from build123d import *

# Parameters (mm, degrees)
F1_DEPTH = 8.3
F2_R     = 1.55
F3_DEPTH = 23.001
F4_R     = 1.55
F5_DEPTH = 16.001
F6_R     = 4.14999


# Not quite as in the source:
# - a fillet or chamfer is up to 0.001 mm smaller than in the source, because OpenCascade refuses the exact size


with BuildPart() as f1:
    # F0 (on Top) → F1 (new body)
    with BuildSketch(Plane.XY):
        Polygon((-57.5197213515, -7.7541078215), (-65.8197213515, -7.7541078215), (-65.8197213515, -14.7041078215), (-49.7500874824, -14.7041078215), (-49.7500874824, -7.7041078215), (-41.4500874824, -7.7041078215), (-41.4500874824, 1.2958921785), (-49.7500874824, 1.2958921785), (-49.7500874824, 8.2958921785), (-65.8197213515, 8.2958921785), (-65.8197213515, 1.3458921785), (-57.5197213515, 1.3458921785), align=None)
    extrude(amount=F1_DEPTH)

    # F2 (on face) → F3 (cut, through all)
    with BuildSketch(Plane.XZ.offset(14.7041078215)):
        with Locations((-61.6697213515, 4.15)):
            Circle(F2_R)
    extrude(amount=-F3_DEPTH, mode=Mode.SUBTRACT)

    # F4 (on face) → F5 (cut, through all)
    with BuildSketch(Plane.XZ.offset(7.7041078215)):
        with Locations((-45.6000874824, 4.15)):
            Circle(F4_R)
    extrude(amount=-F5_DEPTH, mode=Mode.SUBTRACT)

    # F6 (radius 4.15 in the source; OpenCascade refuses exactly that, so slightly less here)
    f6_edges = [f1.edges().sort_by_distance(p)[0] for p in [
        (-65.819721, 4.820892, 8.3),
        (-65.819721, 4.820892, 0),
        (-65.819721, -11.229108, 0),
        (-65.819721, -11.229108, 8.3),
        (-41.450087, -3.204108, 0),
        (-41.450087, -3.204108, 8.3),
    ]]
    fillet(f6_edges, radius=F6_R)


solid = f1.part
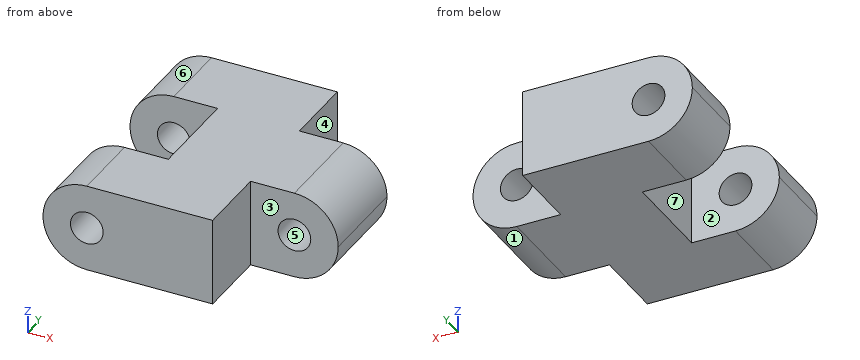
Could you check a few things on this model? Use its own coordinates, in mm. Face numbers are marked on the shaded views. A direction names the side the tool comes from. Coordinates: 2 decimals unless noted, no trailing zeros. Write each loop counter-clockwise with the first axis right and the second up, starting at its lowest first coordinate (ties: lowest second). Pieces come first, ordered by that corner, then holes. Notation, with made-up numbers: (51.5, 59.25) - (79.5, 59.25) arc R24 ccw to (79.5, 69.25) - close; hole circle Ø1 at (88, 62). An arc over 180 degrees is marked (long way). Put each result on its own line as item: value. Start each with the question number.
Q1. I want a section at B-B on z = 5. Write out the boundary of the cut face in (x, y).
Q2. I'm going to push flat-ended pins straight in: P1, Ø2, axis at x = -47, z = 6.5, coming from the -Y side; P2, Ø2.5, axis at x = -47, z = 2.5, coming from the +Y side; P3, Ø1.5, axis at y = 4, z = 6.5, coming from the -X side. Where does each tip first touch, or does it pass through?
Q3. Which directions (+Z, -Z, +X, -X, +Y, -Y) give clear straight access to the entire face, cutting with the end or side of a thin tool? Please do the marked faces 1, 2, 3 and 4.
Q4. I want a section at C-C on x = -62.25. Write out the boundary of the cut face in (y, z), plus the area to 3 significant figures.
Q5. Please list where these lines run through material, in increasing order: L1, parallel to Y at x = -63, z = 2; L2, parallel to X at y = -9, z = 4; L3, parallel to Y at x = -45.75, z = 6.
Q6. I want a section at D-D on x = -44.75. Write out the boundary of the cut face in (y, z), plus the area to 3 significant figures.
Q7. Thinking about a two-plate mould opening in Z: for the marked faces 5, 6 and 7, which applies, pulls with the +Z half, pulls with the -Z half, needs draft (parallel to the pull), parting line crosses it, or undercut?
Checks:
1. outline: (-65.73, -14.7) - (-62.97, -14.7) - (-62.97, -7.75) - (-65.73, -7.75) - close; (-65.73, 1.35) - (-62.97, 1.35) - (-62.97, 8.3) - (-65.73, 8.3) - close; (-60.37, -14.7) - (-49.75, -14.7) - (-49.75, -7.7) - (-46.9, -7.7) - (-46.9, 1.3) - (-49.75, 1.3) - (-49.75, 8.3) - (-60.37, 8.3) - (-60.37, 1.35) - (-57.52, 1.35) - (-57.52, -7.75) - (-60.37, -7.75) - close; (-44.3, -7.7) - (-41.54, -7.7) - (-41.54, 1.3) - (-44.3, 1.3) - close
2. P1: y = -7.7
2. P2: y = 1.3
2. P3: x = -65.5
3. face 1: -Z, +X, +Y, -Y
3. face 2: +Z, -Z, -X
3. face 3: +Z, -Z, +X, -Y
3. face 4: +Z, -Z, +X, +Y
4. outline: (-14.7, 0.04) - (-7.75, 0.04) - (-7.75, 2.71) - (-14.7, 2.71) - close; (-14.7, 5.59) - (-7.75, 5.59) - (-7.75, 8.26) - (-14.7, 8.26) - close; (1.35, 0.04) - (8.3, 0.04) - (8.3, 2.71) - (1.35, 2.71) - close; (1.35, 5.59) - (8.3, 5.59) - (8.3, 8.26) - (1.35, 8.26) - close
4. area: 74.3 mm²
5. L1: -14.7 to -7.75, 1.35 to 8.3
5. L2: -65.82 to -63.21, -60.13 to -49.75
5. L3: -7.7 to 1.3
6. outline: (-7.7, 0.09) - (1.3, 0.09) - (1.3, 2.85) - (-7.7, 2.85) - close; (-7.7, 5.45) - (1.3, 5.45) - (1.3, 8.21) - (-7.7, 8.21) - close
6. area: 49.8 mm²
7. face 5: undercut
7. face 6: pulls with the +Z half
7. face 7: needs draft
